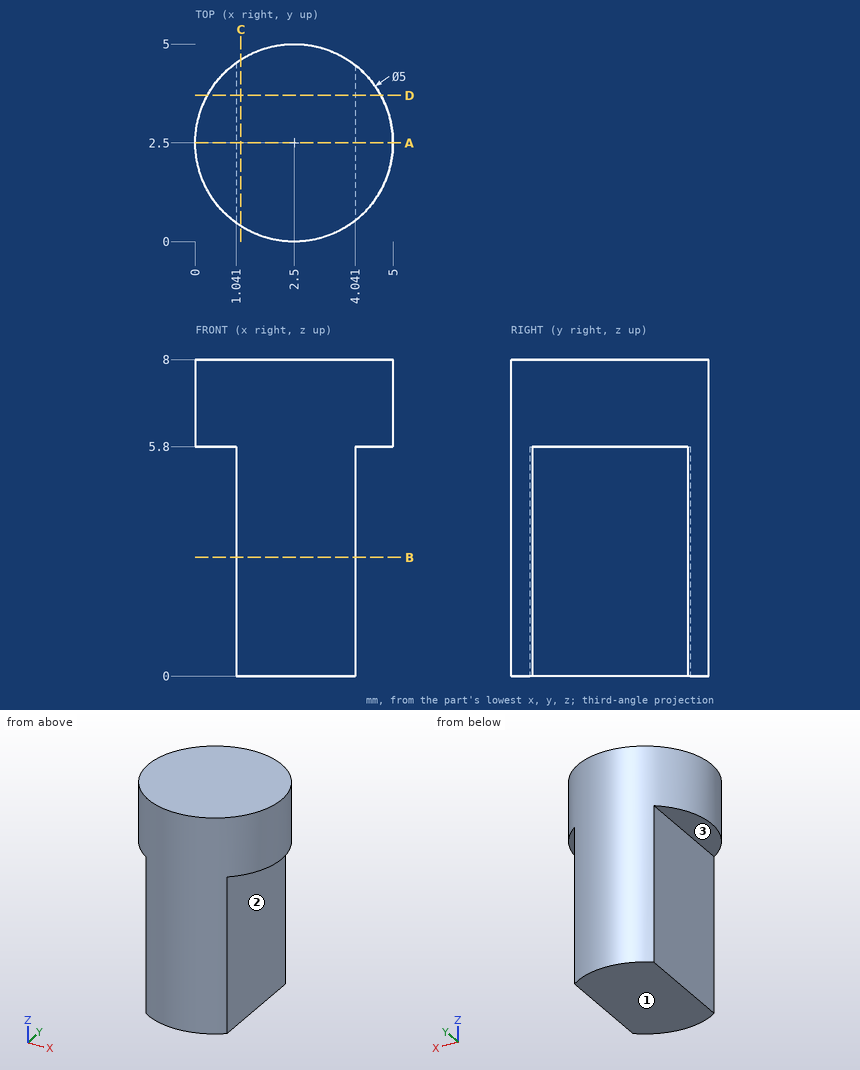
Design review of the part shown in the three views and the two pictorial views. Dimensions are in mm from the part's minimum x, y and z. A direction names the side the tool comes from. Give positions to 0.01 mm unless a question says otherwise; leave off trailing zeros. Write each loop counter-clockwise with the first axis right and the second up, starting at its lowest first coordinate (ties: lowest second). Pieces come first, ordered by that corner, then holes. Notation, with made-up numbers: M 43,22.25 L 51,22.25 A19 ccw 51,38.25 Z; hole C 20.25,55.5 d4. An arc over 180 degrees is marked long. Answer in a Markdown table with one row per item.
Item 1: For P1, Ø2, axis at y = 1.5, z = 3, coming from the +X side; P2, Ø3, axis at y = 3.5, z = 4.5, coming from the -X side, all flat-tipped, find the tip position at first contact; note any pin that passes through.
Check sheet entries:
| item | result |
|---|---|
| P1 | x = 4.04 |
| P2 | x = 0.01 |
Item 2: Tool access review of the marked faces 1, 2 and 3: name each direction out of +Z, -Z, +X, -X, +Y, -Y from which nothing blocks a thin tool from reaching the whole face with its end or side.
Check sheet entries:
| item | result |
|---|---|
| face 1 | -Z, +X, -X, +Y, -Y |
| face 2 | -Z, +X, +Y, -Y |
| face 3 | -Z, -X, +Y, -Y |
Item 3: Add section D-D on y = 3.7. Give the boundary of the cut face in (x, z), plus the area to 4 significant figures.
Check sheet entries:
| item | result |
|---|---|
| outline | M 0.31,5.8 L 1.04,5.8 L 1.04,0 L 4.04,0 L 4.04,5.8 L 4.69,5.8 L 4.69,8 L 0.31,8 Z |
| area | 27.05 mm2 |
Item 4: Add section B-B on z = 3. Give the boundary of the cut face in (x, y).
Check sheet entries:
| item | result |
|---|---|
| outline | M 1.04,0.47 A2.5 ccw 4.04,0.53 L 4.04,4.47 A2.5 ccw 1.04,4.53 Z |
Item 5: Add section A-A on y = 2.5. Give the boundary of the cut face in (x, z).
Check sheet entries:
| item | result |
|---|---|
| outline | M 0,5.8 L 1.04,5.8 L 1.04,0 L 4.04,0 L 4.04,5.8 L 5,5.8 L 5,8 L 0,8 Z |
Item 6: For line 1 along X through (y, z) = (2.7, 5.5); line 2 along Z through (x, y) = (4.5, 3.3); line 3 along Y through (x, z) = (4, 0.5), list the stretches that pass through material, from the lowest coordinate up.
Check sheet entries:
| item | result |
|---|---|
| line 1 | 1.04 to 4.04 |
| line 2 | 5.8 to 8 |
| line 3 | 0.5 to 4.5 |
Item 7: Add section C-C on x = 1.15. Give the boundary of the cut face in (y, z), plus the area to 3 significant figures.
Check sheet entries:
| item | result |
|---|---|
| outline | M 0.4,0 L 4.6,0 L 4.6,8 L 0.4,8 Z |
| area | 33.7 mm2 |
